Check sheet for the modelled part. Datum: model origin and axes. Units: mm. Face numbers are marked on the shaded views. Round coordinates to 2 decimals unless told otherwise and drop trailing zeros. Write each loop counter-clockwise with the first axis right and the second up, starting at its lowest first coordinate (ties: lowest second). Pieces come first, ordered by that corner, then holes. Notation, with made-up numbers: M 41,43 L 87,43 A15 cw 87,59 Z; hole C 34,28.5 d10. An arc over 180 degrees is marked long. Answer in a Markdown table with one row per item.
```python
from build123d import *

# Parameters (mm, degrees)
F0_W     = 2133.6
F0_H     = 365.76
F1_DEPTH = 152.4
F2_T     = -3.048
F3_R     = 152.4
F4_DEPTH = 152.401


with BuildPart() as f1:
    # F0 (on Top) → F1 (new body)
    with BuildSketch(Plane.XY):
        Rectangle(F0_W, F0_H)
    extrude(amount=F1_DEPTH)

    # F2
    f2_openings = [f1.faces().sort_by_distance(p)[0] for p in [
        (0, 0, 0),
    ]]
    offset(amount=F2_T, openings=f2_openings)

    # F3 (on face) → F4 (cut, through all)
    with BuildSketch(Plane.XY.offset(152.4)):
        with Locations((182.88, 0)):
            Circle(F3_R)
        with Locations((518.16, 0)):
            Circle(F3_R)
        with Locations((853.44, 0)):
            Circle(F3_R)
        with Locations((-182.88, 0)):
            Circle(F3_R)
        with Locations((-518.16, 0)):
            Circle(F3_R)
        with Locations((-853.44, 0)):
            Circle(F3_R)
    extrude(amount=-F4_DEPTH, mode=Mode.SUBTRACT)


solid = f1.part
```
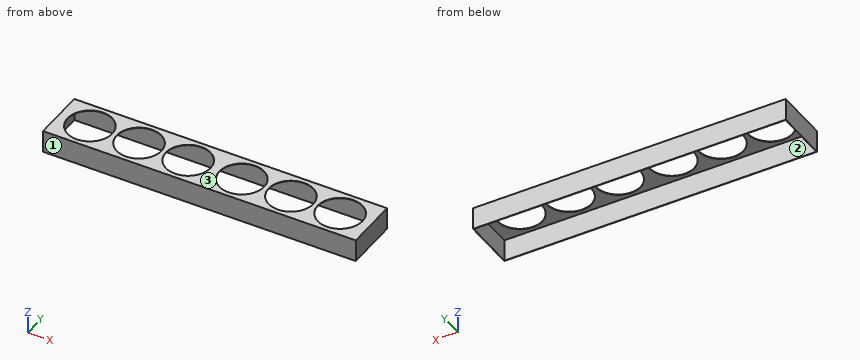
1. Section check C-C, the plane y = -78. Count the separate pieces of the cut face and the enclosed holes in it, and give its area (3 significant figures).
Found:
| item | result |
|---|---|
| separate pieces | 7 |
| enclosed holes | 0 |
| area | 2,620 mm2 |
2. Scan lines: L1, parallel to X at y = 41.5, z = 37; L2, parallel to Y at x = 873, z = 18; L3, parallel to Y at x = -182.88, z = 151.05. Record each from-to range of solid material in increasing order.
Found:
| item | result |
|---|---|
| L1 | x = -1066.8 to -1063.75, 1063.75 to 1066.8 |
| L2 | y = -182.88 to -179.83, 179.83 to 182.88 |
| L3 | y = -182.88 to -152.4, 152.4 to 182.88 |
3. Section check A-A, the plane z = 39. Record the cut outline in (x, y), and give its area (3 significant figures).
Found:
| item | result |
|---|---|
| outline | M -1066.8,-182.88 L 1066.8,-182.88 L 1066.8,182.88 L -1066.8,182.88 Z; hole M -1063.75,-179.83 L 1063.75,-179.83 L 1063.75,179.83 L -1063.75,179.83 Z |
| area | 15,200 mm2 |
4. Draft check along Y on the marked faces 1, 2 and 3. Enter one of: +Y half, -Y half, draft (parallel to the pull), parting line (faces both ways), or undercut.
Found:
| item | result |
|---|---|
| face 1 | -Y half |
| face 2 | undercut |
| face 3 | draft |
5. Section check B-B, the plane x = -853.44. Record the cut outline in (y, z), and give its area (3 significant figures).
Found:
| item | result |
|---|---|
| outline | M -182.88,0 L -179.83,0 L -179.83,149.35 L -152.4,149.35 L -152.4,152.4 L -182.88,152.4 Z; M 152.4,149.35 L 179.83,149.35 L 179.83,0 L 182.88,0 L 182.88,152.4 L 152.4,152.4 Z |
| area | 1,100 mm2 |
